from build123d import *

# Parameters (mm, degrees)
BOSS_EXTRUDE1_DEPTH            = 11.90625
F_5_16_0_3125_DIAMETER_HOLE1_D = 7.9375
SKETCH4_W                      = 635
SKETCH4_H                      = 1212.85
CUT_EXTRUDE1_DEPTH             = 12.90625


with BuildPart() as part:
    # Sketch1 → Boss-Extrude1 (new body)
    with BuildSketch(Plane.XY):
        Polygon((1068.467396061, -524.104266958), (941.467396061, -524.104266958), (941.467396061, -727.304266958), (-201.532603939, -727.304266958), (-201.532603939, -524.104266958), (-328.532603939, -524.104266958), (-328.532603939, 72.795733042), (70.055437863, 485.545733042), (669.87935426, 485.545733042), (1068.467396061, 72.795733042), align=None)
    extrude(amount=BOSS_EXTRUDE1_DEPTH)

    # 5/16 (0.3125) Diameter Hole1 (through all)
    with Locations(Plane.XY.offset(11.90625)):
        with Locations((-303.132603939, 80.815834959), (-138.032603939, 251.781889765), (57.355437863, 454.112130003), (682.57935426, 454.112130003), (877.967396061, 251.781889765), (1043.067396061, 80.815834959)):
            Hole(F_5_16_0_3125_DIAMETER_HOLE1_D / 2)

    # Sketch4 → Cut-Extrude1 (cut, through all)
    with BuildSketch(Plane.XY.offset(11.90625)):
        with Locations((750.967396061, -120.879266958)):
            Rectangle(SKETCH4_W, SKETCH4_H)
    extrude(amount=-CUT_EXTRUDE1_DEPTH, mode=Mode.SUBTRACT)


solid = part.part
Design review of the part built by this model. Coordinates are the model's own, in mm. Round coordinates to 2 decimals unless told otherwise and drop trailing zeros. Order: outer loops, then holes, each group sorted by start corner. A loop starts at its lowest first (then second) coordinate and runs counter-clockwise, first axis right, second up.
1) For L1, parallel to X at y = -668.5, z = 1.5; L2, parallel to Y at x = 27, z = 4.25; L3, parallel to Y at x = 2.5, z = 3.5, list the stretches that pass through material, from the lowest coordinate up.
The answers:
L1: x = -201.53 to 433.47
L2: y = -727.3 to 440.96
L3: y = -727.3 to 415.59
2) Consider section C-C (x = -32). State the section outline as (y, z) points.
The answers:
outline: (-727.3, 0) - (379.86, 0) - (379.86, 11.91) - (-727.3, 11.91) - close
3) Consider section A-A (z = 3). State the section outline as (x, y) points.
The answers:
outline: (-328.53, -524.1) - (-201.53, -524.1) - (-201.53, -727.3) - (433.47, -727.3) - (433.47, 485.55) - (70.06, 485.55) - (-328.53, 72.8) - close; hole circle Ø7.94 at (-303.13, 80.82); hole circle Ø7.94 at (-138.03, 251.78); hole circle Ø7.94 at (57.36, 454.11)
4) Clearance check with flat-ended pins moving along their axes: pin 1 Ø5 at (x, y) = (57.36, 454.11) entering from -Z; pin 2 Ø6 at (x, z) = (-249.5, 3) entering from -Y; pin 3 Ø3.5 at (y, z) = (-620.5, 7) entering from -X; pin 4 Ø6 at (x, z) = (24.5, 8.5) entering from +Y. State where each tip first meets the part, or that it passes through.
The answers:
pin 1: passes through
pin 2: stops at y = -524.1
pin 3: stops at x = -201.53
pin 4: stops at y = 441.48
5) Consider section B-B (y = 168). State the section outline as (x, z) points.
The answers:
outline: (-236.59, 0) - (433.47, 0) - (433.47, 11.91) - (-236.59, 11.91) - close
